Here's how the part is built. I have some questions about the finished solid (model axes, mm). Coordinates: 2 decimals unless noted, no trailing zeros. Write each loop counter-clockwise with the first axis right and the second up, starting at its lowest first coordinate (ties: lowest second). Pieces come first, ordered by that corner, then holes. Notation, with made-up numbers: M -4.5,-30 L 16.5,-30 A18 cw 16.5,-5 Z; hole C -8,7.25 d8. An arc over 180 degrees is marked long. Use one line per item in the form item = value. Start each with the question number.
1. I'm going to push a flat-ended pin straight in: pin 1 Ø3 at (x, y) = (12, 107) entering from -Z. Where does the tip first touch, or does it pass through?
2. Please list where these lines run through material, in increasing order: line 1 along Y through (x, z) = (19, -1.7); line 2 along Y through (x, z) = (6, -1.6); line 3 along Y through (x, z) = (40.5, -1.7). Write a range as [from, to].
3. I want a section at A-A, the plane x = 52.5. List the corners of the cut face in (y, z) for me.
4. I want a section at B-B, the plane z = -0.9. Count the separate pieces of the cut face and the enclosed holes in it, plus the area to 3 significant figures.
5. I want a section at C-C, the plane y = 89. List the corners of the cut face in (x, z) for me, plus the area to 4 significant figures.
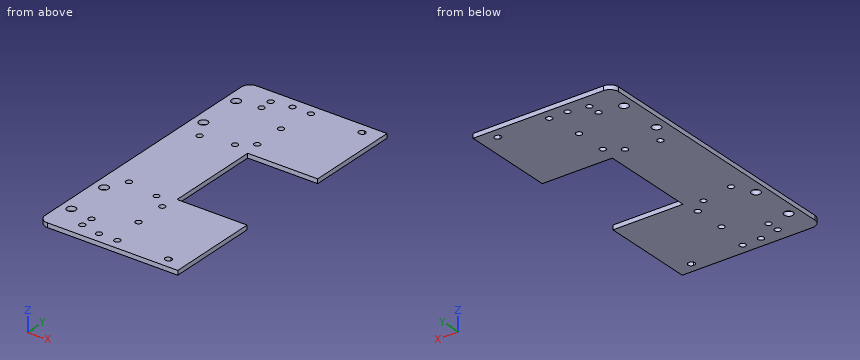
from build123d import *

# Parameters (mm, degrees)
SKETCH_1_W                  = 82
SKETCH_1_H                  = 160
EXTRUDE_1_DEPTH             = 50
SKETCH_2_W                  = 79.5
SKETCH_2_H                  = 47.5
CUT_EXTRUDE_1_DEPTH         = 187.611896727
CUT_EXTRUDE_2_DEPTH         = 186.95765647
CUT_EXTRUDE_4_DEPTH         = 186.95765647
CUT_EXTRUDE_5_DEPTH         = 186.95765647
CUT_EXTRUDE_7_DEPTH         = 186.95765647
CUT_EXTRUDE_9_DEPTH         = 187.611896727
CUT_EXTRUDE_10_DEPTH        = 187.611896727
CUT_EXTRUDE_11_DEPTH        = 187.611896727
CUT_EXTRUDE_12_DEPTH        = 187.611896727
CUT_EXTRUDE_13_DEPTH        = 187.611896727
CUT_EXTRUDE_14_DEPTH        = 187.611896727
CUT_EXTRUDE_15_DEPTH        = 187.611896727
CUT_EXTRUDE_16_DEPTH        = 187.611896727
CUT_EXTRUDE_17_DEPTH        = 187.611896727
CUT_EXTRUDE_18_DEPTH        = 187.611896727
CUT_EXTRUDE_19_DEPTH        = 187.611896727
DRAFT_1_ANGLE               = 30
DRAFT_2_ANGLE               = 30
HOLE_WIZARD_3_2_3_2_1_D     = 3.2
HOLE_WIZARD_3_2_3_2_1_DEPTH = 50
HOLE_WIZARD_3_4_3_4_1_D     = 3.4
HOLE_WIZARD_3_4_3_4_1_DEPTH = 50
HOLE_WIZARD_3_2_3_2_2_D     = 3.2
HOLE_WIZARD_3_2_3_2_2_DEPTH = 82
HOLE_WIZARD_5_0_5_1_D       = 5
HOLE_WIZARD_5_0_5_1_DEPTH   = 50
FILLET_3_R                  = 5
SKETCH_31_W                 = 2.5
SKETCH_31_H                 = 160
CUT_EXTRUDE_21_DEPTH        = 10
SKETCH_32_R                 = 1.7
CUT_EXTRUDE_22_DEPTH        = 10
SKETCH_33_R                 = 1.7
CUT_EXTRUDE_23_DEPTH        = 10
SKETCH_34_W                 = 60.596480557
SKETCH_34_H                 = 37.741752596
SKETCH_34_W_2               = 35.854664966
SKETCH_34_H_2               = 6.290292099
SKETCH_34_W_3               = 37.951428999
SKETCH_34_H_3               = 7.758026922
SKETCH_34_W_4               = 17.193465071
SKETCH_34_H_4               = 10.693496569
SKETCH_34_W_5               = 15.306377442
SKETCH_34_H_5               = 12.999937006
EXTRUDE_2_DEPTH             = 2.5
SKETCH_35_W                 = 40
SKETCH_35_H                 = 27
CUT_EXTRUDE_24_DEPTH        = 179.679881352
SKETCH_37_R                 = 1.7
CUT_EXTRUDE_25_DEPTH        = 10


with BuildPart() as part:
    # 草图1 → 凸台-拉伸1 (new body)
    with BuildSketch(Plane(origin=(0, 0, -50), x_dir=(-1, 0, 0), z_dir=(0, 0, -1))):
        with Locations((-41, 80)):
            Rectangle(SKETCH_1_W, SKETCH_1_H)
    extrude(amount=-EXTRUDE_1_DEPTH)

    # 草图2 → 切除-拉伸1 (cut, through all)
    with BuildSketch(Plane(origin=(0, 160, 0), x_dir=(-1, 0, 0), z_dir=(0, 1, 0))):
        with Locations((-39.75, -26.25)):
            Rectangle(SKETCH_2_W, SKETCH_2_H)
    extrude(amount=-CUT_EXTRUDE_1_DEPTH, mode=Mode.SUBTRACT)

    # 草图3 → 切除-拉伸2 (cut, through all)
    with BuildSketch(Plane(origin=(0, 0, -2.5), x_dir=(-1, 0, 0), z_dir=(0, 0, -1))):
        with BuildLine():
            Line((-65, 89.5), (-20, 89.5))
            ThreePointArc((-20, 89.5), (-17.5, 92), (-20, 94.5))
            Line((-20, 94.5), (-65, 94.5))
            ThreePointArc((-65, 94.5), (-67.5, 92), (-65, 89.5))
        make_face()
    extrude(amount=-CUT_EXTRUDE_2_DEPTH, mode=Mode.SUBTRACT)

    # 草图5 → 切除-拉伸4 (cut, through all)
    with BuildSketch(Plane(origin=(0, 0, -2.5), x_dir=(-1, 0, 0), z_dir=(0, 0, -1))):
        with BuildLine():
            Line((-65, 65.5), (-20, 65.5))
            ThreePointArc((-20, 65.5), (-17.5, 68), (-20, 70.5))
            Line((-20, 70.5), (-65, 70.5))
            ThreePointArc((-65, 70.5), (-67.5, 68), (-65, 65.5))
        make_face()
    extrude(amount=-CUT_EXTRUDE_4_DEPTH, mode=Mode.SUBTRACT)

    # 草图6 → 切除-拉伸5 (cut, through all)
    with BuildSketch(Plane(origin=(0, 0, -2.5), x_dir=(-1, 0, 0), z_dir=(0, 0, -1))):
        with BuildLine():
            Line((-68, 50), (-38, 50))
            ThreePointArc((-38, 50), (-36.4, 51.6), (-38, 53.2))
            Line((-38, 53.2), (-68, 53.2))
            ThreePointArc((-68, 53.2), (-69.6, 51.6), (-68, 50))
        make_face()
    extrude(amount=-CUT_EXTRUDE_5_DEPTH, mode=Mode.SUBTRACT)

    # 草图8 → 切除-拉伸7 (cut, through all)
    with BuildSketch(Plane(origin=(0, 0, -2.5), x_dir=(-1, 0, 0), z_dir=(0, 0, -1))):
        with BuildLine():
            Line((-68, 106.8), (-38, 106.8))
            ThreePointArc((-38, 106.8), (-36.4, 108.4), (-38, 110))
            Line((-38, 110), (-68, 110))
            ThreePointArc((-68, 110), (-69.6, 108.4), (-68, 106.8))
        make_face()
    extrude(amount=-CUT_EXTRUDE_7_DEPTH, mode=Mode.SUBTRACT)

    # 草图10 → 切除-拉伸9 (cut, through all)
    with BuildSketch(Plane(origin=(82, 0, 0), x_dir=(0, 0, -1), z_dir=(1, 0, 0))):
        with BuildLine():
            Line((20.690598923, 80), (16.690598923, 86.92820323))
            ThreePointArc((16.690598923, 86.92820323), (13.629378785, 80), (16.690598923, 73.07179677))
            Line((16.690598923, 73.07179677), (20.690598923, 80))
        make_face()
    extrude(amount=-CUT_EXTRUDE_9_DEPTH, mode=Mode.SUBTRACT)

    # 草图11 → 切除-拉伸10 (cut, through all)
    with BuildSketch(Plane(origin=(82, 0, 0), x_dir=(0, 0, -1), z_dir=(1, 0, 0))):
        with BuildLine():
            Line((24.154700538, 89.29920473), (24.154700538, 82))
            Line((24.154700538, 82), (32.154700538, 82))
            ThreePointArc((32.154700538, 82), (29.315895428, 86.922283358), (24.154700538, 89.29920473))
        make_face()
    extrude(amount=-CUT_EXTRUDE_10_DEPTH, mode=Mode.SUBTRACT)

    # 草图12 → 切除-拉伸11 (cut, through all)
    with BuildSketch(Plane(origin=(82, 0, 0), x_dir=(0, 0, -1), z_dir=(1, 0, 0))):
        with BuildLine():
            Line((24.154700538, 78), (24.154700538, 70.70079527))
            ThreePointArc((24.154700538, 70.70079527), (29.315895428, 73.077716642), (32.154700538, 78))
            Line((32.154700538, 78), (24.154700538, 78))
        make_face()
    extrude(amount=-CUT_EXTRUDE_11_DEPTH, mode=Mode.SUBTRACT)

    # 草图13 → 切除-拉伸12 (cut, through all)
    with BuildSketch(Plane(origin=(82, 0, 0), x_dir=(0, 0, -1), z_dir=(1, 0, 0))):
        with BuildLine():
            Line((36, 21.2), (14, 21.2))
            ThreePointArc((14, 21.2), (12.4, 19.6), (14, 18))
            Line((14, 18), (36, 18))
            ThreePointArc((36, 18), (37.6, 19.6), (36, 21.2))
        make_face()
    extrude(amount=-CUT_EXTRUDE_12_DEPTH, mode=Mode.SUBTRACT)

    # 草图14 → 切除-拉伸13 (cut, through all)
    with BuildSketch(Plane(origin=(82, 0, 0), x_dir=(0, 0, -1), z_dir=(1, 0, 0))):
        with BuildLine():
            Line((36, 31.2), (14, 31.2))
            ThreePointArc((14, 31.2), (12.4, 29.6), (14, 28))
            Line((14, 28), (36, 28))
            ThreePointArc((36, 28), (37.6, 29.6), (36, 31.2))
        make_face()
    extrude(amount=-CUT_EXTRUDE_13_DEPTH, mode=Mode.SUBTRACT)

    # 草图15 → 切除-拉伸14 (cut, through all)
    with BuildSketch(Plane(origin=(82, 0, 0), x_dir=(0, 0, -1), z_dir=(1, 0, 0))):
        with BuildLine():
            Line((36, 41.2), (14, 41.2))
            ThreePointArc((14, 41.2), (12.4, 39.6), (14, 38))
            Line((14, 38), (36, 38))
            ThreePointArc((36, 38), (37.6, 39.6), (36, 41.2))
        make_face()
    extrude(amount=-CUT_EXTRUDE_14_DEPTH, mode=Mode.SUBTRACT)

    # 草图16 → 切除-拉伸15 (cut, through all)
    with BuildSketch(Plane(origin=(82, 0, 0), x_dir=(0, 0, -1), z_dir=(1, 0, 0))):
        with BuildLine():
            Line((36, 51.2), (14, 51.2))
            ThreePointArc((14, 51.2), (12.4, 49.6), (14, 48))
            Line((14, 48), (36, 48))
            ThreePointArc((36, 48), (37.6, 49.6), (36, 51.2))
        make_face()
    extrude(amount=-CUT_EXTRUDE_15_DEPTH, mode=Mode.SUBTRACT)

    # 草图17 → 切除-拉伸16 (cut, through all)
    with BuildSketch(Plane(origin=(82, 0, 0), x_dir=(0, 0, -1), z_dir=(1, 0, 0))):
        with BuildLine():
            Line((36, 112), (14, 112))
            ThreePointArc((14, 112), (12.4, 110.4), (14, 108.8))
            Line((14, 108.8), (36, 108.8))
            ThreePointArc((36, 108.8), (37.6, 110.4), (36, 112))
        make_face()
    extrude(amount=-CUT_EXTRUDE_16_DEPTH, mode=Mode.SUBTRACT)

    # 草图18 → 切除-拉伸17 (cut, through all)
    with BuildSketch(Plane(origin=(82, 0, 0), x_dir=(0, 0, -1), z_dir=(1, 0, 0))):
        with BuildLine():
            Line((36, 122), (14, 122))
            ThreePointArc((14, 122), (12.4, 120.4), (14, 118.8))
            Line((14, 118.8), (36, 118.8))
            ThreePointArc((36, 118.8), (37.6, 120.4), (36, 122))
        make_face()
    extrude(amount=-CUT_EXTRUDE_17_DEPTH, mode=Mode.SUBTRACT)

    # 草图19 → 切除-拉伸18 (cut, through all)
    with BuildSketch(Plane(origin=(82, 0, 0), x_dir=(0, 0, -1), z_dir=(1, 0, 0))):
        with BuildLine():
            Line((36, 132), (14, 132))
            ThreePointArc((14, 132), (12.4, 130.4), (14, 128.8))
            Line((14, 128.8), (36, 128.8))
            ThreePointArc((36, 128.8), (37.6, 130.4), (36, 132))
        make_face()
    extrude(amount=-CUT_EXTRUDE_18_DEPTH, mode=Mode.SUBTRACT)

    # 草图20 → 切除-拉伸19 (cut, through all)
    with BuildSketch(Plane(origin=(82, 0, 0), x_dir=(0, 0, -1), z_dir=(1, 0, 0))):
        with BuildLine():
            Line((36, 142), (14, 142))
            ThreePointArc((14, 142), (12.4, 140.4), (14, 138.8))
            Line((14, 138.8), (36, 138.8))
            ThreePointArc((36, 138.8), (37.6, 140.4), (36, 142))
        make_face()
    extrude(amount=-CUT_EXTRUDE_19_DEPTH, mode=Mode.SUBTRACT)

    # 拔模1
    draft_1_faces = [part.faces().sort_by_distance(p)[0] for p in [
        (80.75, 85.649602365, -24.154700538),
    ]]
    draft(draft_1_faces, Plane(origin=(0, 82, -24.154700538), x_dir=(0, 0, 1), z_dir=(0, 1, 0)), DRAFT_1_ANGLE)

    # 拔模2
    draft_2_faces = [part.faces().sort_by_distance(p)[0] for p in [
        (80.75, 74.350397635, -24.154700538),
    ]]
    draft(draft_2_faces, Plane(origin=(0, 78, -32.154700538), x_dir=(0, 0, -1), z_dir=(0, -1, 0)), DRAFT_2_ANGLE)

    # Ø3.2 (3.2) 直径孔1
    with Locations(Plane.XY):
        with Locations((30, 32.75), (30, 38.75), (30, 50)):
            Hole(HOLE_WIZARD_3_2_3_2_1_D / 2, depth=HOLE_WIZARD_3_2_3_2_1_DEPTH)

    # Ø3.4 (3.4) 直径孔1
    with Locations(Plane.XY):
        with Locations((30, 154), (40.5, 154), (69.5, 154), (69.5, 6), (40.5, 6), (30, 6), (30, 121.25), (30, 127.25), (30, 110), (19, 8), (19, 15), (19, 145), (12, 53), (12, 107), (19, 152), (22, 124.25), (22, 35.75)):
            Hole(HOLE_WIZARD_3_4_3_4_1_D / 2, depth=HOLE_WIZARD_3_4_3_4_1_DEPTH)

    # Ø3.2 (3.2) 直径孔2
    with Locations(Plane(origin=(82, 0, 0), x_dir=(0, 0, -1), z_dir=(1, 0, 0))):
        with Locations((9.5, 150), (17.5, 150), (25.5, 150), (33.5, 150), (41.5, 150), (41.5, 10), (33.5, 10), (25.5, 10), (17.5, 10), (10.5, 90), (23, 100), (35.5, 90), (9.5, 10), (35.5, 70), (23, 60), (10.5, 70)):
            Hole(HOLE_WIZARD_3_2_3_2_2_D / 2, depth=HOLE_WIZARD_3_2_3_2_2_DEPTH)

    # Ø5.0 (5) 直径孔1
    with Locations(Plane.XY):
        with Locations((6, 17), (6, 42), (6, 118), (6, 143)):
            Hole(HOLE_WIZARD_5_0_5_1_D / 2, depth=HOLE_WIZARD_5_0_5_1_DEPTH)

    # 圆角3
    fillet_3_edges = [part.edges().sort_by_distance(p)[0] for p in [
        (80.75, 160, -50),
        (80.75, 0, -50),
        (0, 160, -1.25),
        (0, 0, -1.25),
    ]]
    fillet(fillet_3_edges, radius=FILLET_3_R)

    # 草图31 → 切除-拉伸21 (cut)
    with BuildSketch(Plane.ZY.offset(-79.5)):
        with Locations((-1.25, 80)):
            Rectangle(SKETCH_31_W, SKETCH_31_H)
    extrude(amount=-CUT_EXTRUDE_21_DEPTH, mode=Mode.SUBTRACT)


with BuildPart() as body_2:
    # of the pieces the cut leaves, the one that is kept (cut_extrude_21_keep)
    add(part.part.solids().sort_by_distance((5, 160, -2.5))[0])

    # 草图32 → 切除-拉伸22 (cut)
    with BuildSketch(Plane.XY):
        with Locations((38, 25.5)):
            Circle(SKETCH_32_R)
        with Locations((38, 43.7)):
            Circle(SKETCH_32_R)
    extrude(amount=-CUT_EXTRUDE_22_DEPTH, mode=Mode.SUBTRACT)

    # 草图33 → 切除-拉伸23 (cut)
    with BuildSketch(Plane.XY):
        with Locations((38, 134.5)):
            Circle(SKETCH_33_R)
        with Locations((38, 116.3)):
            Circle(SKETCH_33_R)
    extrude(amount=-CUT_EXTRUDE_23_DEPTH, mode=Mode.SUBTRACT)

    # 草图34 → 凸台-拉伸2 (add)
    with BuildSketch(Plane.XY):
        with Locations((44.153204469, 79.233741422)):
            Rectangle(SKETCH_34_W, SKETCH_34_H)
        with Locations((52.540260602, 108.378761482)):
            Rectangle(SKETCH_34_W_2, SKETCH_34_H_2)
        with Locations((53.588642619, 51.032265177)):
            Rectangle(SKETCH_34_W_3, SKETCH_34_H_3)
        with Locations((26.016195584, 35.096858526)):
            Rectangle(SKETCH_34_W_4, SKETCH_34_H_4)
        with Locations((26.959739398, 123.47546252)):
            Rectangle(SKETCH_34_W_5, SKETCH_34_H_5)
    extrude(amount=-EXTRUDE_2_DEPTH)

    # 草图35 → 切除-拉伸24 (cut, through all)
    with BuildSketch(Plane.XY):
        Polygon((79.5, 64.187810857), (79.5, 80), (39.5, 80), (39.5, 53), (79.5, 53), align=None)
        with Locations((59.5, 93.5)):
            Rectangle(SKETCH_35_W, SKETCH_35_H)
    extrude(amount=-CUT_EXTRUDE_24_DEPTH, mode=Mode.SUBTRACT)

    # 草图37 → 切除-拉伸25 (cut)
    with BuildSketch(Plane.XY):
        with Locations((70, 6)):
            Circle(SKETCH_37_R)
        with Locations((70, 154)):
            Circle(SKETCH_37_R)
    extrude(amount=-CUT_EXTRUDE_25_DEPTH, mode=Mode.SUBTRACT)


solid = body_2.part
Answer list:
q1.pin_1 = through
q2.line_1 = [0, 6.3], [9.7, 13.3], [16.7, 143.3], [146.7, 150.3], [153.7, 160]
q2.line_2 = [0, 14.5], [19.5, 39.5], [44.5, 115.5], [120.5, 140.5], [145.5, 160]
q2.line_3 = [0, 4.3], [7.7, 53], [107, 152.3], [155.7, 160]
q3.outline = M 0,-2.5 L 53,-2.5 L 53,0 L 0,0 Z; M 107,-2.5 L 160,-2.5 L 160,0 L 107,0 Z
q4.separate_pieces = 1
q4.enclosed_holes = 22
q4.area = 10,300 mm²
q5.outline = M 0,-2.5 L 39.5,-2.5 L 39.5,0 L 0,0 Z
q5.area = 98.75 mm²
